```python
from build123d import *

# Parameters (mm, degrees)
SKETCH_1_W               = 70.6
SKETCH_1_H               = 84.6
EXTRUDE_1_DEPTH          = 23
SKETCH_2_W               = 18
SKETCH_2_H               = 4.7
EXTRUDE_2_DEPTH          = 2
SKETCH_3_W               = 70.6
SKETCH_3_H               = 3.2
EXTRUDE_3_DEPTH          = 10
CUT_EXTRUDE_START        = -2
SKETCH_4_R               = 11
CUT_EXTRUDE_1_DEPTH      = 115.979827321
EXTRUDE_START            = -2
EXTRUDE_1_2_DEPTH        = 2
DELETE_START             = 107
DELETE_FACE_1_DEPTH      = 2
CUT_EXTRUDE_2_DEPTH      = 1
CUT_EXTRUDE_2_DEPTH_BACK = 43
CUT_EXTRUDE_2_START      = -2
EXTRUDE_START_2          = 24
EXTRUDE_4_DEPTH          = 2
FILLET_1_R               = 5
FILLET_2_R               = 3.5
FILLET_3_R               = 3.5


# Read off the part's stored shape, not the designer's step: 删除面1
with BuildPart() as part:
    # 草图1 → Extrude 1 (new body)
    with BuildSketch(Plane.XY):
        with Locations((38.5, 152.5)):
            Rectangle(SKETCH_1_W, SKETCH_1_H)
    extrude(amount=-EXTRUDE_1_DEPTH)

    # 草图2 → 凸台-拉伸2 (add)
    with BuildSketch(Plane(origin=(0, 0, -23), x_dir=(-1, 0, 0), z_dir=(0, 0, -1))):
        with Locations((-12.2, 197.15)):
            Rectangle(SKETCH_2_W, SKETCH_2_H)
        with Locations((-64.8, 197.15)):
            Rectangle(SKETCH_2_W, SKETCH_2_H)
    extrude(amount=-EXTRUDE_2_DEPTH)

    # 草图3 → 凸台-拉伸3 (add)
    with BuildSketch(Plane(origin=(0, 0, -23), x_dir=(-1, 0, 0), z_dir=(0, 0, -1))):
        with Locations((-38.5, 108.6)):
            Rectangle(SKETCH_3_W, SKETCH_3_H)
    extrude(amount=-EXTRUDE_3_DEPTH)

    # 草图4 → 切除-拉伸1 (cut, through all)
    with BuildSketch(Plane(origin=(0, 194.8, 0), x_dir=(1, 0, 0), z_dir=(0, 1, 0)).offset(CUT_EXTRUDE_START)):
        with Locations((60.8, 25)):
            Circle(SKETCH_4_R)
    extrude(amount=-CUT_EXTRUDE_1_DEPTH, mode=Mode.SUBTRACT)

    # 草图5 → Extrude 1 2 (add)
    with BuildSketch(Plane.XZ.offset(-107).offset(EXTRUDE_START)):
        with BuildLine():
            ThreePointArc((71.616653826, -23), (60.8, -14), (49.983346174, -23))
            Line((49.983346174, -23), (51.950010506, -23.363636364))
            ThreePointArc((51.950010506, -23.363636364), (60.8, -16), (69.649989494, -23.363636364))
            Line((69.649989494, -23.363636364), (71.616653826, -23))
        make_face()
    extrude(amount=EXTRUDE_1_2_DEPTH)

    # Delete Face 1 outline → Delete Face 1 (cut)
    with BuildSketch(Plane(origin=(0, 0, 0), x_dir=(1, 0, 0), z_dir=(0, 1, 0)).offset(DELETE_START)):
        with BuildLine():
            Line((49.983346174, 23), (52.025035613, 23))
            ThreePointArc((52.025035613, 23), (51.985647631, 23.181431245), (51.950010506, 23.363636364))
            Line((51.950010506, 23.363636364), (49.983346174, 23))
        make_face()
        with BuildLine():
            Line((71.616653826, 23), (69.649989494, 23.363636364))
            ThreePointArc((69.649989494, 23.363636364), (69.614352369, 23.181431245), (69.574964387, 23))
            Line((69.574964387, 23), (71.616653826, 23))
        make_face()
    extrude(amount=DELETE_FACE_1_DEPTH, mode=Mode.SUBTRACT)

    # 草图6 → 切除-拉伸2 (cut, two sides: drawn at the far end of the back side and taken through both)
    with BuildSketch(Plane.ZY.offset(-3.2).offset(CUT_EXTRUDE_2_START - CUT_EXTRUDE_2_DEPTH_BACK)):
        Polygon((-23, 107), (-15, 107), (-15, 112.2), (-2, 112.2), (-2, 192.8), (-23, 192.8), align=None)
    extrude(amount=CUT_EXTRUDE_2_DEPTH + CUT_EXTRUDE_2_DEPTH_BACK, mode=Mode.SUBTRACT)

    # 草图7 → 凸台-拉伸4 (add)
    with BuildSketch(Plane(origin=(4.2, 0, 0), x_dir=(0, 0, -1), z_dir=(1, 0, 0)).offset(EXTRUDE_START_2)):
        Polygon((23, 107), (23, 192.8), (2, 192.8), (2, 112.2), (15, 112.2), (15, 107), align=None)
    extrude(amount=EXTRUDE_4_DEPTH)

    # 圆角1
    fillet_1_edges = [part.edges().sort_by_distance(p)[0] for p in [
        (71.687482194, 107, -23),
        (50.112517807, 107, -23),
        (29.2, 107, -23),
        (3.7, 107, -23),
    ]]
    fillet(fillet_1_edges, radius=FILLET_1_R)

    # 圆角2
    fillet_2_edges = [part.edges().sort_by_distance(p)[0] for p in [
        (73.8, 194.8, -10.5),
        (3.2, 194.8, -10.5),
        (3.2, 110.2, -6.5),
        (73.8, 110.2, -6.5),
    ]]
    fillet(fillet_2_edges, radius=FILLET_2_R)

    # 圆角3
    fillet_3_edges = [part.edges().sort_by_distance(p)[0] for p in [
        (39.2, 192.8, -2),
        (39.2, 112.2, -2),
        (28.2, 192.8, -12.5),
        (28.2, 152.5, -2),
        (28.2, 112.2, -8.5),
        (30.2, 192.8, -12.5),
        (30.2, 152.5, -2),
        (30.2, 112.2, -8.5),
        (48.2, 112.2, -8.5),
        (16.2, 112.2, -2),
        (48.2, 152.5, -2),
        (16.2, 192.8, -2),
        (48.2, 192.8, -12.5),
        (4.2, 112.2, -8.5),
        (4.2, 152.5, -2),
        (4.2, 192.8, -12.5),
    ]]
    fillet(fillet_3_edges, radius=FILLET_3_R)


solid = part.part
```
Input: part model. Units: mm. Frame: model coordinates. A direction names the side the tool comes from. Coordinates: 2 decimals unless noted, no trailing zeros. Loops run counter-clockwise (first coordinate to the right, second up) from the corner with the lowest first, then second, coordinate; pieces in that order, holes last. Notation, with made-up numbers: M -31.5,10.25 L 24.5,10.25 A23 ccw 24.5,47.25 Z; hole C -8.5,74 d3. An arc over 180 degrees is marked long. One line per item, written item: value.
(1) Pull-direction query (X, two-part tool) for faces 5 (the cylindrical face through (47.2, 153.02, -3.05)), 6 (the cylindrical face through (39.12, 191.75, -3)), 7 (the cylindrical face through (72.8, 111.25, -6.59)), 8 (the flat face through (39, 108, -13)); classes: +X half, -X half, draft (parallel to the pull), parting line (faces both ways), or undercut.
Filled in:
face 5: undercut
face 6: undercut
face 7: +X half
face 8: draft
(2) Line query: line 1 along X through (y, z) = (119, -7.5); line 2 along X through (y, z) = (135, -18); line 3 along X through (y, z) = (151.5, -17.75). Output: solid intervals per line, ascending. Write a range as from..to.
Filled in:
line 1: 3.2..4.2, 28.2..30.2, 48.2..73.8
line 2: 3.2..4.2, 28.2..30.2, 48.2..52.31, 69.29..73.8
line 3: 3.2..4.2, 28.2..30.2, 48.2..52.53, 69.07..73.8
(3) Section D-D (x = 40.5). Output: boundary loops of the cut face in (y, z).
Filled in:
outline: M 107,-15 L 112.2,-15 L 112.2,-5.5 A3.5 cw 115.7,-2 L 189.3,-2 A3.5 cw 192.8,-5.5 L 192.8,-23 L 194.8,-23 L 194.8,0 L 110.2,0 L 110.2,-13 L 107,-13 Z
(4) Section A-A (z = -11.25). Output: boundary loops of the cut face in (x, y).
Filled in:
outline: M 3.2,113.7 A3.5 ccw 6.7,110.2 L 70.3,110.2 A3.5 ccw 73.8,113.7 L 73.8,191.3 A3.5 ccw 70.3,194.8 L 6.7,194.8 A3.5 ccw 3.2,191.3 Z; hole M 4.2,115.7 A3.5 ccw 7.7,112.2 L 24.7,112.2 A3.5 ccw 28.2,115.7 L 28.2,189.3 A3.5 ccw 24.7,192.8 L 7.7,192.8 A3.5 ccw 4.2,189.3 Z; hole M 30.2,115.7 A3.5 ccw 33.7,112.2 L 44.7,112.2 A3.5 ccw 48.2,115.7 L 48.2,189.3 A3.5 ccw 44.7,192.8 L 33.7,192.8 A3.5 ccw 30.2,189.3 Z
(5) Pin query (flat end, axial travel): pin 1 (2 mm diameter, centred on x = 52, z = -20, fed in from -Y); pin 2 (7 mm diameter, centred on x = 13, y = 111, fed in from -Z); pin 3 (1 mm diameter, centred on x = 49.5, z = -10, fed in from -Y). Return the tip coordinate at first contact, or that it passes through.
Filled in:
pin 1: y = 107.1
pin 2: z = -15
pin 3: y = 110.2
(6) Reachability of faces 1 (the flat face through (3.2, 153, -12)), 2 (the flat face through (21.2, 197, -22)), 3 (the cylindrical face through (4.2, 111.25, -6.59)), 4 (the flat face through (4.2, 149, -14)) from +Z, -Z, +X, -X, +Y, -Y: full face, straight path, thin tool, end or side. Return the list, or none.
Filled in:
face 1: +Z, -Z, -X, +Y, -Y
face 2: +Z, -Z, +Y
face 3: +Z, -X, -Y
face 4: -Z
(7) Section B-B (x = 13). Output: boundary loops of the cut face in (y, z).
Filled in:
outline: M 107,-15 L 112.2,-15 L 112.2,-5.5 A3.5 cw 115.7,-2 L 189.3,-2 A3.5 cw 192.8,-5.5 L 192.8,-23 L 199.5,-23 L 199.5,-21 L 194.8,-21 L 194.8,0 L 110.2,0 L 110.2,-13 L 107,-13 Z
(8) Section C-C (y = 143). Output: boundary loops of the cut face in (x, z).
Filled in:
outline: M 3.2,-23 L 4.2,-23 L 4.2,-5.5 A3.5 cw 7.7,-2 L 24.7,-2 A3.5 cw 28.2,-5.5 L 28.2,-23 L 30.2,-23 L 30.2,-5.5 A3.5 cw 33.7,-2 L 44.7,-2 A3.5 cw 48.2,-5.5 L 48.2,-23 L 49.98,-23 A11 cw 71.62,-23 L 73.8,-23 L 73.8,0 L 3.2,0 Z
